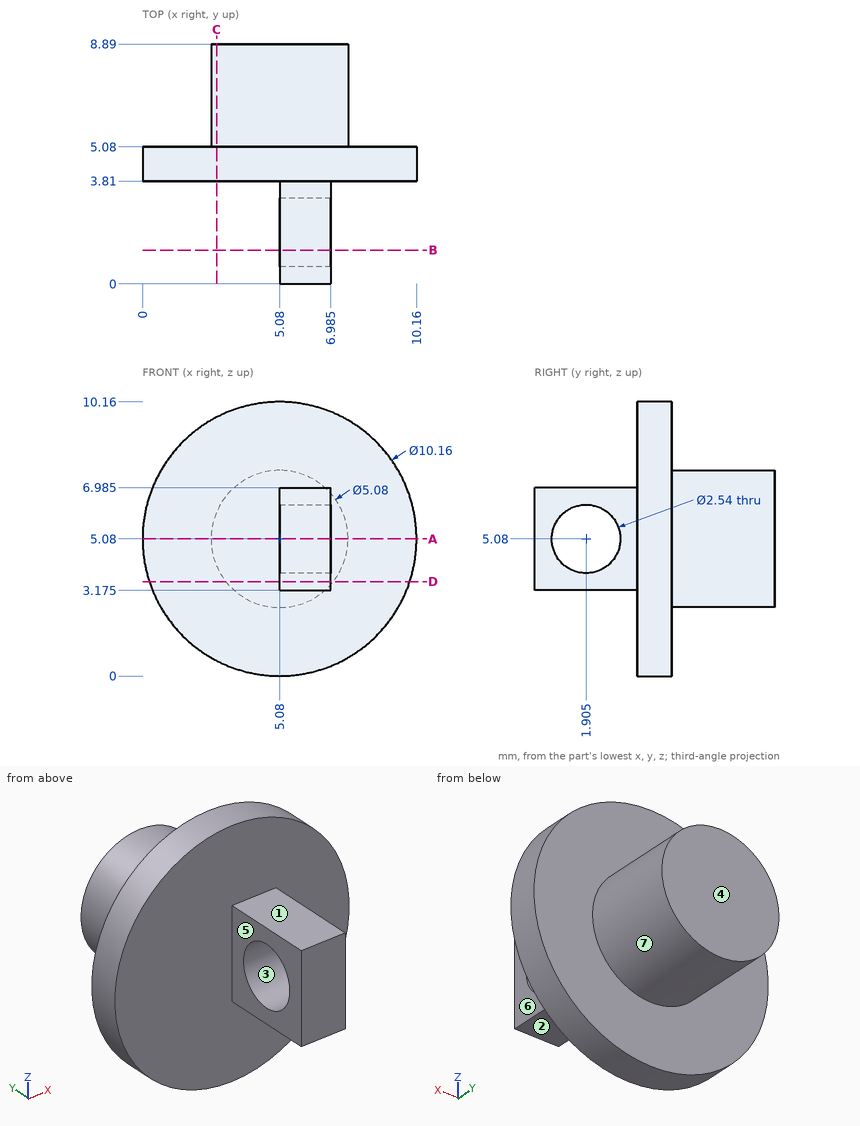
Input: dimensioned drawing with shaded views. Units: mm. Origin: part minimum x, y, z. A direction names the side the tool comes from. Give positions to 0.01 mm unless a question says otherwise; leave off trailing zeros. Loops run counter-clockwise (first coordinate to the right, second up) from the corner with the lowest first, then second, coordinate; pieces in that order, holes last. Notation, with made-up numbers: (-17, 34.5) - (39, 34.5) arc R19 ccw to (39, 45.5) - close; hole circle Ø5 at (89, -13). An arc over 180 degrees is marked (long way). Answer as CSV lines item,"result". Start each with the question number.
(1) Section query C-C (x = 2.75). Output: boundary loops of the cut face in (y, z).
(2) Ray query, line 1 along Y through (x, z) = (6.45, 5.08) (3 decimals); line 2 along Y through (x, z) = (2, 2.5); line 3 along Y through (x, z) = (6.25, 4.25). Return the intervals inside material, ascending. Write a range as [from, to].
(3) Reachability of the marked faces 5, 6 and 7 from +Z, -Z, +X, -X, +Y, -Y: full face, straight path, thin tool, end or side. Return the list, or none.
(4) Section query D-D (z = 3.5). Output: boundary loops of the cut face in (x, y) (3 decimals).
(5) Pin query (flat end, axial travel): P1, Ø1, axis at x = 6.5, y = 2, coming from the +Z side (3 decimals); P2, Ø1.1, axis at y = 1.5, z = 6, coming from the -X side; P3, Ø1.5, axis at x = 2.5, z = 8.5, coming from the -Y side; P4, Ø2, axis at y = 1.905, z = 5.08, coming from the -X side. Return the tip coordinate at first contact, or that it passes through.
(6) Section query A-A (z = 5.08). Output: boundary loops of the cut face in (x, y) (3 decimals), and give its area (3 significant figures).
(7) Mould query, pull axis Z, two halves, no side actions, for the marked faces 1, 2, 3 and 4. Classes: +Z half, -Z half, draft (parallel to the pull), parting line (faces both ways), or undercut.
(8) Section query B-B (y = 1.25). Output: boundary loops of the cut face in (x, z) (3 decimals).
Worked answers:
1,outline,"(3.81, 0.57) - (5.08, 0.57) - (5.08, 4.07) - (8.89, 4.07) - (8.89, 6.09) - (5.08, 6.09) - (5.08, 9.59) - (3.81, 9.59) - close"
2,line 1,"y = [0, 0.635], [3.175, 8.89]"
2,line 2,"y = [3.81, 5.08]"
2,line 3,"y = [0, 0.94], [2.87, 8.89]"
3,face 5,"+Z, -Z, -X, -Y"
3,face 6,"+Z, -Z, +X, -Y"
3,face 7,"+Y"
4,outline,"(0.252, 3.81) - (5.08, 3.81) - (5.08, 0) - (6.985, 0) - (6.985, 3.81) - (9.908, 3.81) - (9.908, 5.08) - (7.069, 5.08) - (7.069, 8.89) - (3.091, 8.89) - (3.091, 5.08) - (0.252, 5.08) - close"
5,P1,"stops at z = 6.985"
5,P2,"stops at x = 5.08"
5,P3,"stops at y = 3.81"
5,P4,"passes through"
6,outline,"(0, 3.81) - (5.08, 3.81) - (5.08, 3.175) - (6.985, 3.175) - (6.985, 3.81) - (10.16, 3.81) - (10.16, 5.08) - (7.62, 5.08) - (7.62, 8.89) - (2.54, 8.89) - (2.54, 5.08) - (0, 5.08) - close; (5.08, 0) - (6.985, 0) - (6.985, 0.635) - (5.08, 0.635) - close"
6,area,"34.7 mm^2"
7,face 1,"+Z half"
7,face 2,"-Z half"
7,face 3,"undercut"
7,face 4,"draft"
8,outline,"(5.08, 3.175) - (6.985, 3.175) - (6.985, 3.992) - (5.08, 3.992) - close; (5.08, 6.168) - (6.985, 6.168) - (6.985, 6.985) - (5.08, 6.985) - close"
